Model file for the job. Use its own axes, mm. Give positions to 0.01 mm unless a question says otherwise; leave off trailing zeros. Use a Markdown table: item, result.
from build123d import *
from build123d.topology import SkipClean

# Parameters (mm, degrees)
SKETCH1_R           = 2.25
BOSS_EXTRUDE1_DEPTH = 6
CHAMFER1_SIZE       = 2.5
CHAMFER2_SIZE       = 2


with BuildPart() as part:
    # Sketch1 → Boss-Extrude1 (new body)
    with BuildSketch(Plane(origin=(0, 0, 0), x_dir=(1, 0, 0), z_dir=(0, 1, 0))):
        with BuildLine():
            Line((265, -131.75), (265, 0))
            Line((265, 0), (0, 0))
            Line((0, 0), (0, -140))
            Line((0, -140), (265, -140))
            Line((265, -140), (265, -136.25))
            ThreePointArc((265, -136.25), (262.75, -134), (265, -131.75))
        make_face()
        with Locations(Location((6, -26.8, 0), (0, 0, 270))):
            Circle(SKETCH1_R, mode=Mode.SUBTRACT)
        with Locations(Location((6, -80.4, 0), (0, 0, 270))):
            Circle(SKETCH1_R, mode=Mode.SUBTRACT)
        with Locations(Location((6, -134, 0), (0, 0, 270))):
            Circle(SKETCH1_R, mode=Mode.SUBTRACT)
        with Locations(Location((57.8, -134, 0), (0, 0, 270))):
            Circle(SKETCH1_R, mode=Mode.SUBTRACT)
        with Locations(Location((109.6, -134, 0), (0, 0, 270))):
            Circle(SKETCH1_R, mode=Mode.SUBTRACT)
        with Locations(Location((161.4, -134, 0), (0, 0, 270))):
            Circle(SKETCH1_R, mode=Mode.SUBTRACT)
        with Locations(Location((213.2, -134, 0), (0, 0, 270))):
            Circle(SKETCH1_R, mode=Mode.SUBTRACT)
    extrude(amount=BOSS_EXTRUDE1_DEPTH)

    # Chamfer1
    chamfer1_edges = [part.edges().sort_by_distance(p)[0] for p in [
        (262.75, 6, 134),
        (57.8, 6, 131.75),
        (109.6, 6, 131.75),
        (6, 6, 131.75),
        (6, 6, 78.15),
        (6, 6, 24.55),
        (213.2, 6, 131.75),
        (161.4, 6, 131.75),
    ]]
    chamfer(chamfer1_edges, length=CHAMFER1_SIZE)

    # Mirror3: part across plane


with BuildPart() as part_1:
    with SkipClean():  # the faces are left unmerged after this step: merging them gives an invalid solid
        add(part.part)
        add(part.part.mirror(Plane(origin=(265, 6, 131.75), x_dir=(0, 0, 1), z_dir=(-1, 0, 0))))

    # Mirror4: part across plane


with BuildPart() as part_2:
    with SkipClean():  # the faces are left unmerged after this step: merging them gives an invalid solid
        add(part_1.part)
        add(part_1.part.mirror(Plane(origin=(0, 6, 0), x_dir=(1, 0, 0), z_dir=(0, 0, -1))))

    # Chamfer2
    chamfer2_edges = [part_2.edges().sort_by_distance(p)[0] for p in [
        (0, 3, 140),
        (530, 3, -140),
        (0, 3, -140),
        (530, 3, 140),
    ]]
    chamfer(chamfer2_edges, length=CHAMFER2_SIZE)


solid = part_2.part
(1) Drill centre lines: probe 1 along Z at (x, y) = (472.2, 2.45); probe 2 along X at (y, z) = (1.5, -26.8); probe 3 along Z at (x, y) = (215, 4.8). Where is each one in solid material? Low to high. Write a range as [from, to].
Computed:
| item | result |
|---|---|
| probe 1 | [-140, -136.25], [-131.75, 131.75], [136.25, 140] |
| probe 2 | [0, 3.75], [8.25, 521.75], [526.25, 530] |
| probe 3 | [-140, -137.06], [-130.94, 130.94], [137.06, 140] |
(2) Pin check, flat tips, straight feed: P1, Ø5, axis at x = 472.2, z = -134, coming from the +Y side; P2, Ø7, axis at x = 6, z = -26.8, coming from the +Y side. Stop position of each tip, or through.
Computed:
| item | result |
|---|---|
| P1 | y = 3.75 |
| P2 | y = 4.75 |
(3) Mould opens along X. For faces 1 (the conical face through (526.349, 3.656, 26.278)), 2 (the flat face through (269, 6, 2)) say: pulls with the +X half, pulls with the -X half, needs draft (parallel to the pull), parting line crosses it, or undercut.
Computed:
| item | result |
|---|---|
| face 1 | undercut |
| face 2 | needs draft |
